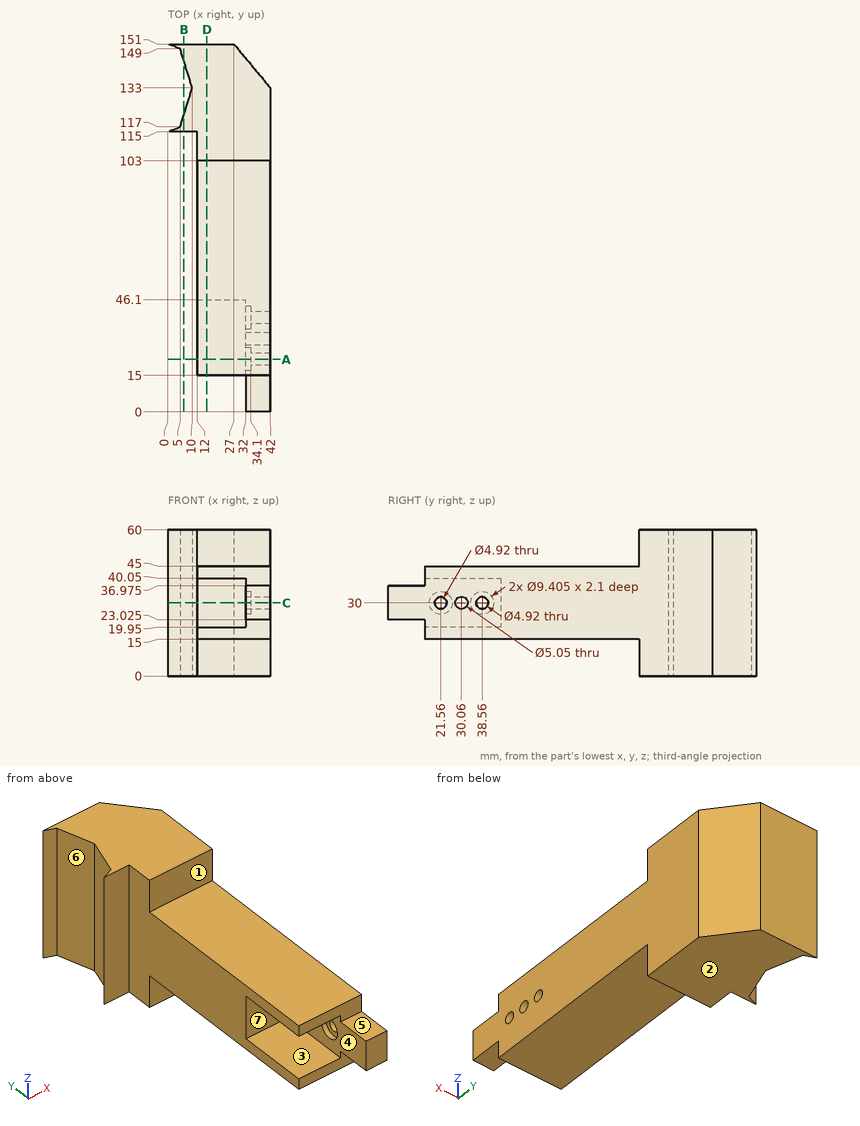
Input: dimensioned drawing with shaded views. Units: mm. Origin: part minimum x, y, z. A direction names the side the tool comes from. Give positions to 0.01 mm unless a question says otherwise; leave off trailing zeros. Order: outer loops, then holes, each group sorted by start corner. A loop starts at its lowest first (then second) coordinate and runs counter-clockwise, first axis right, second up. Notation, with made-up numbers: (64.25, 76) -> (106.25, 76) arc R25 ccw to (106.25, 106) -> close; hole circle Ø11 at (51, 40). An arc over 180 degrees is marked (long way). Answer as a JSON object with one key per item and string values.
Q1. Access query for the marked faces 5, 6 and 7. Directions: +Z, -Z, +X, -X, +Y, -Y. A direction counts if a zero-diameter tool reaches every point of the face in a straight line with its end or side. Return the directions, or none.
Entries:
{"face 5": "+Z, +X, -X, -Y", "face 6": "+Z, -Z, -X", "face 7": "-X, -Y"}
Q2. Section D-D (x = 16). Output: boundary loops of the cut face in (y, z), plus the area to 3 significant figures.
Entries:
{"outline": "(15, 15) -> (103, 15) -> (103, 0) -> (151, 0) -> (151, 60) -> (103, 60) -> (103, 45) -> (15, 45) -> (15, 40.05) -> (46.1, 40.05) -> (46.1, 19.95) -> (15, 19.95) -> close", "area": "4,890 mm^2"}
Q3. Draft query along Z for the marked faces 1, 2, 3 and 4. Return one class per face: released by +Z, released by -Z, zero draft, split by the parting line, or undercut.
Entries:
{"face 1": "zero draft", "face 2": "released by -Z", "face 3": "undercut", "face 4": "undercut"}
Q4. First-contact query: pin 1 (6 mm diameter, centred on x = 23.5, y = 36.5, fed in from -Z); pin 2 (4.5 mm diameter, centred on x = 30.5, z = 54.5, fed in from -Y); pin 3 (4 mm diameter, centred on y = 29.5, z = 40, fed in from -X). Flat tips, straight axial feed; report the tip coordinate or a pass-through.
Entries:
{"pin 1": "stops at z = 15", "pin 2": "stops at y = 103", "pin 3": "stops at x = 12"}
Q5. Section B-B (x = 6.5). Output: boundary loops of the cut face in (y, z), plus the area to 3 significant figures.
Entries:
{"outline": "(115, 0) -> (121.8, 0) -> (121.8, 60) -> (115, 60) -> close; (144.2, 0) -> (151, 0) -> (151, 60) -> (144.2, 60) -> close", "area": "816 mm^2"}
Q6. Material intervals for probe 1 along Y at (x, z) = (33, 30) (1 decimal); probe 2 along Y at (x, z) = (38, 30) (3 decimals); probe 3 along Z at (x, y) = (38.25, 21.56), sorted ascending.
Entries:
{"probe 1": "y = 0 to 16.9, 26.3 to 27.5, 32.6 to 33.9, 43.3 to 143.8", "probe 2": "y = 0 to 19.1, 24.02 to 27.535, 32.585 to 36.1, 41.02 to 137.8", "probe 3": "z = 15 to 27.54, 32.46 to 45"}
Q7. Section A-A (y = 21.56). Output: boundary loops of the cut face in (x, z), plus the area to 3 significant figures.
Entries:
{"outline": "(12, 15) -> (42, 15) -> (42, 27.54) -> (34.1, 27.54) -> (34.1, 25.3) -> (32, 25.3) -> (32, 19.95) -> (12, 19.95) -> close; (12, 40.05) -> (32, 40.05) -> (32, 34.7) -> (34.1, 34.7) -> (34.1, 32.46) -> (42, 32.46) -> (42, 45) -> (12, 45) -> close", "area": "439 mm^2"}
Q8. Section C-C (z = 30). State how many separate pieces and enclosed holes the cut face has, plus the area to 3 significant figures.
Entries:
{"separate pieces": "4", "enclosed holes": "0", "area": "3,490 mm^2"}
